Part model, mm, in its own coordinate system. A direction names the side the tool comes from. Coordinates: 2 decimals unless noted, no trailing zeros. Write each loop counter-clockwise with the first axis right and the second up, starting at its lowest first coordinate (ties: lowest second). Pieces come first, ordered by that corner, then holes. Notation, with made-up numbers: (-30, 86) - (-8, 86) arc R34 ccw to (-8, 120) - close; hole circle Ø6 at (-30.75, 72). An arc over 180 degrees is marked (long way). Write each question's results on one line, items separated by ' | '.
from build123d import *

# Parameters (mm, degrees)
CROQUIS1_W              = 564
CROQUIS1_H              = 724
CROQUIS1_W_2            = 560
CROQUIS1_H_2            = 720
SALIENTE_EXTRUIR1_DEPTH = 20
CROQUIS2_W              = 20
CROQUIS2_H              = 357.467498219
CROQUIS2_W_2            = 271.273547015
CROQUIS2_H_2            = 20
CROQUIS2_W_3            = 268.726452985
CROQUIS2_H_3            = 342.532501781
SALIENTE_EXTRUIR4_DEPTH = 20
CROQUIS4_R              = 7.807995064
SALIENTE_EXTRUIR5_DEPTH = 177


with BuildPart() as part:
    # Croquis1 → Saliente-Extruir1 (new body)
    with BuildSketch(Plane(origin=(0, 0, 0), x_dir=(1, 0, 0), z_dir=(0, 1, 0))):
        with Locations((10.666666667, -90.666666667)):
            Rectangle(CROQUIS1_W, CROQUIS1_H)
        with Locations((10.666666667, -90.666666667)):
            Rectangle(CROQUIS1_W_2, CROQUIS1_H_2, mode=Mode.SUBTRACT)
    extrude(amount=SALIENTE_EXTRUIR1_DEPTH)

    # Croquis2 → Saliente-Extruir4 (add)
    with BuildSketch(Plane(origin=(0, 20, 0), x_dir=(1, 0, 0), z_dir=(0, 1, 0))):
        with Locations((11.940213682, -271.932917557)):
            Rectangle(CROQUIS2_W, CROQUIS2_H)
        with Locations((-133.696559826, -83.199168448)):
            Rectangle(CROQUIS2_W_2, CROQUIS2_H_2)
        with Locations((156.303440174, -83.199168448)):
            Rectangle(CROQUIS2_W_3, CROQUIS2_H_2)
        with Locations((11.940213682, 98.067082443)):
            Rectangle(CROQUIS2_W, CROQUIS2_H_3)
        with Locations((11.940213682, -83.199168448)):
            Rectangle(CROQUIS2_W, CROQUIS2_H_2)
    extrude(amount=-SALIENTE_EXTRUIR4_DEPTH)

    # Croquis4 → Saliente-Extruir5 (add)
    with BuildSketch(Plane.XZ):
        with Locations(Location((279.95622774, 83.01742746, 0), (0, 0, 90))):
            Circle(CROQUIS4_R)
        with Locations(Location((12.04565938, 440.740646454, 0), (0, 0, 90))):
            Circle(CROQUIS4_R)
        with Locations(Location((12.04565938, -258.363567648, 0), (0, 0, 90))):
            Circle(CROQUIS4_R)
        with Locations(Location((-258.982651015, 83.01742746, 0), (0, 0, 90))):
            Circle(CROQUIS4_R)
    extrude(amount=SALIENTE_EXTRUIR5_DEPTH)


solid = part.part
(1) 3-axis set-ups, long thin cutter, end or side, ignore diameter. For faces 4 (the flat face through (-136, 10, 73.199)), 5 (the cylindrical face through (16.797, -87.261, 434.544)), 6 (the flat face through (-271.333, 10, 96)): which of +Z, -Z, +X, -X, +Y, -Y reach the whole face in a straight line?
Return value:
face 4: +Y, -Y | face 5: -Y | face 6: +Z, -Z, -X, +Y, -Y
(2) Flat gauge pin, fed straight in: P1, Ø10, axis at x = -44, z = 80, coming from the -Y side. Where does the tip first touch, or does it go through?
Return value:
P1: stops at y = 0
(3) Two-plate mould, pull along X, no slides. Class faces 1 (the cylindrical face through (16.797, -87.261, -264.56)), 2 (the flat face through (280, -177, 83)), 3 (the flat face through (290.667, 10, -96)): released by +X, released by -X, zero draft, split by the parting line, or undercut.
Return value:
face 1: split by the parting line | face 2: zero draft | face 3: undercut
(4) Wall check: line 1 (Z direction, x = -240, y = 10.5). Give the ranges that are in metal, low to high. Write a range as from..to.
Return value:
line 1: z = -271.33..-269.33, 73.2..93.2, 450.67..452.67
(5) Saw through at C-C on y = -110.5. Write the cut outline in (x, z), then the cut area to 3 significant figures.
Return value:
outline: circle Ø15.62 at (-258.98, 83.02); circle Ø15.62 at (12.05, -258.36); circle Ø15.62 at (12.05, 440.74); circle Ø15.62 at (279.96, 83.02) | area: 766 mm^2
(6) Saw through at B-B on z = 302. Write the cut outline in (x, y).
Return value:
outline: (-271.33, 0) - (-269.33, 0) - (-269.33, 20) - (-271.33, 20) - close; (1.94, 0) - (21.94, 0) - (21.94, 20) - (1.94, 20) - close; (290.67, 0) - (292.67, 0) - (292.67, 20) - (290.67, 20) - close
(7) Saw through at A-A on x = 219. Write the cut outline in (y, z).
Return value:
outline: (0, -271.33) - (20, -271.33) - (20, -269.33) - (0, -269.33) - close; (0, 73.2) - (20, 73.2) - (20, 93.2) - (0, 93.2) - close; (0, 450.67) - (20, 450.67) - (20, 452.67) - (0, 452.67) - close
